Build history of the part. All positions in model axes, mm. Face numbers are marked on the shaded views. A direction names the side the tool comes from. Round coordinates to 2 decimals unless told otherwise and drop trailing zeros. Loops run counter-clockwise (first coordinate to the right, second up) from the corner with the lowest first, then second, coordinate; pieces in that order, holes last. Notation, with made-up numbers: M -37,54 L -25,54 A24 ccw -25,91 Z; hole C 41,2 d6. An arc over 180 degrees is marked long. One line per item, written item: value.
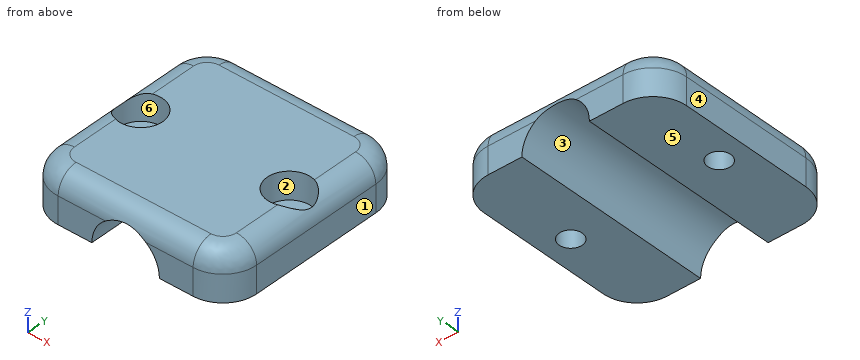
```python
from build123d import *

# Parameters (mm, degrees)
F0_W           = 30
F0_H           = 30
F1_DEPTH       = 7
F3_D           = 3.4
F3_CBORE_D     = 6.5
F3_CBORE_DEPTH = 4
F5_DEPTH       = 30
F6_R           = 5
F7_T1_DEPTH    = 20
F7_T3_DEPTH    = 20
F7_T6_ANGLE    = 90
F7_T8_ANGLE    = 90
F7_T10_ANGLE   = 90
F7_T12_ANGLE   = 90


# Not quite as in the source:
# - a fillet or chamfer that OpenCascade refuses, or shapes differently, is made with other operations: its cross-section is extruded or revolved along the edge and cut away or added


with BuildPart() as f1:
    # F0 (on Top) → F1 (new body)
    with BuildSketch(Plane.XY):
        Rectangle(F0_W, F0_H)
    extrude(amount=F1_DEPTH)

    # F3 (through all)
    with Locations(Plane.XY.offset(7)):
        with Locations((-11, 0), (11, 0)):
            CounterBoreHole(F3_D / 2, F3_CBORE_D / 2, F3_CBORE_DEPTH)

    # F4 (on face) → F5 (cut, through all)
    with BuildSketch(Plane.XZ.offset(15)):
        with BuildLine():
            Line((-5, 0), (5, 0))
            ThreePointArc((5, 0), (0, 5), (-5, 0))
        make_face()
    extrude(amount=-F5_DEPTH, mode=Mode.SUBTRACT)

    # F6
    f6_edges = [f1.edges().sort_by_distance(p)[0] for p in [
        (15, -15, 3.5),
        (-15, -15, 3.5),
        (15, 15, 3.5),
        (-15, 15, 3.5),
    ]]
    fillet(f6_edges, radius=F6_R)

    # F7: fillet of radius 3 on 8 edges, made by hand

    # F7_s2 → F7_t1 (cut)
    with BuildSketch(Plane.YZ.offset(-10)):
        with BuildLine():
            ThreePointArc((-15, 4), (-14.1213203436, 6.1213203436), (-12, 7))
            Line((-12, 7), (-15, 7))
            Line((-15, 7), (-15, 4))
        make_face()
        with BuildLine():
            ThreePointArc((12, 7), (14.1213203436, 6.1213203436), (15, 4))
            Line((15, 4), (15, 7))
            Line((15, 7), (12, 7))
        make_face()
    extrude(amount=F7_T1_DEPTH, mode=Mode.SUBTRACT)

    # F7_s4 → F7_t3 (cut)
    with BuildSketch(Plane.XZ.offset(-10)):
        with BuildLine():
            ThreePointArc((-12, 7), (-14.1213203436, 6.1213203436), (-15, 4))
            Line((-15, 4), (-15, 7))
            Line((-15, 7), (-12, 7))
        make_face()
        with BuildLine():
            ThreePointArc((12, 7), (14.1213203436, 6.1213203436), (15, 4))
            Line((15, 4), (15, 7))
            Line((15, 7), (12, 7))
        make_face()
    extrude(amount=F7_T3_DEPTH, mode=Mode.SUBTRACT)

    # F7_s5 → F7_t6 (revolve, cut)
    with BuildSketch(Plane.YZ.offset(-10)):
        with BuildLine():
            ThreePointArc((-15, 4), (-14.1213203436, 6.1213203436), (-12, 7))
            Line((-12, 7), (-15, 7))
            Line((-15, 7), (-15, 4))
        make_face()
    revolve(axis=Axis((-10, -10, 7), (0, 0, -1)), revolution_arc=F7_T6_ANGLE, mode=Mode.SUBTRACT)

    # F7_s7 → F7_t8 (revolve, cut)
    with BuildSketch(Plane.YZ.offset(10)):
        with BuildLine():
            ThreePointArc((-12, 7), (-14.1213203436, 6.1213203436), (-15, 4))
            Line((-15, 4), (-15, 7))
            Line((-15, 7), (-12, 7))
        make_face()
    revolve(axis=Axis((10, -10, 7), (0, 0, 1)), revolution_arc=F7_T8_ANGLE, mode=Mode.SUBTRACT)

    # F7_s9 → F7_t10 (revolve, cut)
    with BuildSketch(Plane.XZ.offset(-10)):
        with BuildLine():
            ThreePointArc((-12, 7), (-14.1213203436, 6.1213203436), (-15, 4))
            Line((-15, 4), (-15, 7))
            Line((-15, 7), (-12, 7))
        make_face()
    revolve(axis=Axis((-10, 10, 7), (0, 0, -1)), revolution_arc=F7_T10_ANGLE, mode=Mode.SUBTRACT)

    # F7_s11 → F7_t12 (revolve, cut)
    with BuildSketch(Plane.XZ.offset(-10)):
        with BuildLine():
            ThreePointArc((12, 7), (14.1213203436, 6.1213203436), (15, 4))
            Line((15, 4), (15, 7))
            Line((15, 7), (12, 7))
        make_face()
    revolve(axis=Axis((10, 10, 7), (0, 0, 1)), revolution_arc=F7_T12_ANGLE, mode=Mode.SUBTRACT)


solid = f1.part
```
Item 1: Drop flat-ended pins along their axis: P1, Ø2, axis at y = -10.5, z = 2, coming from the +X side; P2, Ø2, axis at x = -12, y = 1, coming from the +Z side; P3, Ø2.5, axis at x = -11, y = 0, coming from the -Z side. Give the stop position or say it passes through.
Check values:
P1: stops at x = 15
P2: stops at z = 3
P3: passes through
Item 2: Slice it at C-C, the plane x = -5.5. Give the cut face in (y, z).
Check values:
outline: M -15,0 L 15,0 L 15,4 A3 ccw 12,7 L -12,7 A3 ccw -15,4 Z
Item 3: Pull direction X, two halves, no side cores. Call the marked faces 3, 4, 5 and 6: pulls with the +X half, pulls with the -X half, needs draft (parallel to the pull), parting line crosses it, or undercut.
Check values:
face 3: undercut
face 4: pulls with the -X half
face 5: needs draft
face 6: undercut
Item 4: Slice it at D-D, the plane y = 7.5. Give the cut face in (x, z), and give its area (3 significant figures).
Check values:
outline: M -15,0 L -5,0 A5 cw 5,0 L 15,0 L 15,4 A3 ccw 12,7 L -12,7 A3 ccw -15,4 Z
area: 167 mm2
Item 5: Slice it at A-A, the plane z = 2. Give the cut face in (x, y), and give its area (3 significant figures).
Check values:
outline: M -15,-10 A5 ccw -10,-15 L -4.58,-15 L -4.58,15 L -10,15 A5 ccw -15,10 Z; M 4.58,-15 L 10,-15 A5 ccw 15,-10 L 15,10 A5 ccw 10,15 L 4.58,15 Z; hole C -11,0 d3.4; hole C 11,0 d3.4
area: 585 mm2
Item 6: Wall check: line 1 along X through (y, z) = (-2.5, 6.5); line 2 along X through (y, z) = (0, 5.6); line 3 along X through (y, z) = (0, 4.5). Give the ranges that are in metal, low to high.
Check values:
line 1: x = -13.66 to -13.08, -8.92 to 8.92, 13.08 to 13.66
line 2: x = -14.54 to -14.25, -7.75 to 7.75, 14.25 to 14.54
line 3: x = -14.96 to -14.25, -7.75 to -2.18, 2.18 to 7.75, 14.25 to 14.96
Item 7: Slice it at B-B, the plane y = 0. Give the cut face in (x, z).
Check values:
outline: M -15,0 L -12.7,0 L -12.7,3 L -14.25,3 L -14.25,5.98 A3 ccw -15,4 Z; M -9.3,0 L -5,0 A5 cw 5,0 L 9.3,0 L 9.3,3 L 7.75,3 L 7.75,7 L -7.75,7 L -7.75,3 L -9.3,3 Z; M 12.7,0 L 15,0 L 15,4 A3 ccw 14.25,5.98 L 14.25,3 L 12.7,3 Z
Item 8: Which spindle directions (+Z, -Z, +X, -X, +Y, -Y) get a long thin tool onto all of the face, cutting with end or side? Do the marked faces 1 and 2. Say none if no direction does.
Check values:
face 1: +Z, -Z, +X, +Y, -Y
face 2: +Z
